Input: part model. Units: mm. Frame: model coordinates. Coordinates: 2 decimals unless noted, no trailing zeros.
1) Section query A-A (y = -0.85). State how many separate pieces and enclosed holes the cut face has, then the cut area to 3 significant figures.
2) Line query: L1, parallel to X at y = -0.9, z = -38. Output: solid intervals per line, ascending.
3) Draft query along X for faces 1 (the cylindrical face through (0.167, -0.493, -25.178)), 2 (the flat face through (-1, -1, 17)). Return one class per face: pulls with the +X half, pulls with the -X half, needs draft (parallel to the pull), parting line crosses it, or undercut.
from build123d import *

# Parameters (mm, degrees)
F0_W     = 101.6
F0_H     = 139.7
F0_W_2   = 40.132
F0_H_2   = 1.524
F0_W_3   = 73.66
F0_W_4   = 6.35
F0_H_3   = 2.286
F1_DEPTH = 1


with BuildPart() as f1:
    # F0 (on Front) → F1 (new body)
    with BuildSketch(Plane.XZ):
        Rectangle(F0_W, F0_H)
        with Locations((-23.114, -57.854202)):
            Rectangle(F0_W_2, F0_H_2, mode=Mode.SUBTRACT)
        Polygon((-36.83, -61.156202), (0, -61.156202), (36.83, -61.156202), (36.83, -62.680202), (0, -62.680202), (-36.83, -62.680202), align=None, mode=Mode.SUBTRACT)
        Polygon((-36.829936, -53.036838), (0, -52.968277), (36.829936, -53.036838), (36.827099, -54.560835), (0, -54.49228), (-36.827099, -54.560835), align=None, mode=Mode.SUBTRACT)
        with Locations((-23.114, -49.666277)):
            Rectangle(F0_W_2, F0_H_2, mode=Mode.SUBTRACT)
        Polygon((-43.18, -42.336936), (-43.18, -40.812936), (-3.048, -40.812936), (-3.048, -42.336936), (-43.18, -42.411644), align=None, mode=Mode.SUBTRACT)
        with Locations((0, -45.602277)):
            Rectangle(F0_W_3, F0_H_2, mode=Mode.SUBTRACT)
        with Locations((0, -37.510936)):
            Rectangle(F0_W_3, F0_H_2, mode=Mode.SUBTRACT)
        with BuildLine():
            ThreePointArc((14.359987, -20.186644), (-0.050304, -25.178638), (-14.460596, -20.186644))
            Line((-14.460596, -20.186644), (14.359987, -20.186644))
        make_face(mode=Mode.SUBTRACT)
        with Locations((-23.114, -2.794)):
            Rectangle(F0_W_2, F0_H_2, mode=Mode.SUBTRACT)
        Polygon((40.132, -7.62), (0, -7.62), (-40.132, -7.62), (-40.132, -6.096), (0, -6.096), (40.132, -6.096), align=None, mode=Mode.SUBTRACT)
        with Locations((23.114, -57.854202)):
            Rectangle(F0_W_2, F0_H_2, mode=Mode.SUBTRACT)
        with Locations((23.114, -49.666277)):
            Rectangle(F0_W_2, F0_H_2, mode=Mode.SUBTRACT)
        Polygon((3.048, -40.812936), (43.18, -40.812936), (43.18, -42.411644), (3.048, -42.336936), align=None, mode=Mode.SUBTRACT)
        with Locations((23.114, -2.794)):
            Rectangle(F0_W_2, F0_H_2, mode=Mode.SUBTRACT)
        Polygon((40.132, 0.508), (0, 0.508), (-40.132, 0.508), (-40.132, 2.032), (0, 2.032), (40.132, 2.032), align=None, mode=Mode.SUBTRACT)
        with Locations((-9.525, 14.46316)):
            Rectangle(F0_W_4, F0_H_3, mode=Mode.SUBTRACT)
        with Locations((-9.525, 23.09916)):
            Rectangle(F0_W_4, F0_H_3, mode=Mode.SUBTRACT)
        with Locations((-9.525, 31.73516)):
            Rectangle(F0_W_4, F0_H_3, mode=Mode.SUBTRACT)
        with Locations((-23.114, 49.276)):
            Rectangle(F0_W_2, F0_H_2, mode=Mode.SUBTRACT)
        with Locations((-23.114, 57.404)):
            Rectangle(F0_W_2, F0_H_2, mode=Mode.SUBTRACT)
        Polygon((-40.132, 54.102), (0, 54.102), (40.132, 54.102), (40.132, 52.578), (0, 52.578), (-40.132, 52.578), align=None, mode=Mode.SUBTRACT)
        Polygon((-40.132, 62.23), (0, 62.23), (40.132, 62.23), (40.132, 60.706), (0, 60.706), (-40.132, 60.706), align=None, mode=Mode.SUBTRACT)
        with Locations((9.525, 14.46316)):
            Rectangle(F0_W_4, F0_H_3, mode=Mode.SUBTRACT)
        with Locations((9.525, 23.09916)):
            Rectangle(F0_W_4, F0_H_3, mode=Mode.SUBTRACT)
        with Locations((9.525, 31.73516)):
            Rectangle(F0_W_4, F0_H_3, mode=Mode.SUBTRACT)
        with Locations((23.114, 49.276)):
            Rectangle(F0_W_2, F0_H_2, mode=Mode.SUBTRACT)
        with Locations((23.114, 57.404)):
            Rectangle(F0_W_2, F0_H_2, mode=Mode.SUBTRACT)
    extrude(amount=F1_DEPTH)


solid = f1.part
Answer:
1. separate pieces: 1
1. enclosed holes: 27
1. area: 12,300 mm2
2. L1: x = -50.8 to -36.83, 36.83 to 50.8
3. face 1: undercut
3. face 2: needs draft
